Read the model definition and answer for the solid it produces. Units are mm, in the model's axes. Face numbers are marked on the shaded views. A direction names the side the tool comes from. Give positions to 0.01 mm unless a question says otherwise; leave off trailing zeros. Write each loop counter-clockwise with the first axis right and the second up, starting at its lowest first coordinate (ties: lowest second). Pieces come first, ordered by that corner, then holes. Notation, with made-up numbers: M 77.25,8.5 L 119.25,8.5 A13 cw 119.25,27.5 Z; hole C 76,26 d3. An arc over 180 degrees is marked long. Use a Markdown table: item, result. Add a question column.
Item 1: A cutting plane is placed at B-B on x = -7.25. Determine the outline of the cut face in (y, z).
Item 2: Consider probe 1 along Z at (x, y) = (-10.5, 37); probe 2 along X at (y, z) = (36, -1.25); probe 3 along Y at (x, z) = (-5.5, 0.5). Determine where each line is inside the solid, lowest interval first. Write a range as [from, to].
Item 3: A cutting plane is placed at D-D on z = -2.7. Determine the outline of the cut face in (x, y).
Item 4: For the marked faces 1, 2 and 3, determine the directions among +Z, -Z, +X, -X, +Y, -Y from which every point of the face is accessible in a straight line to the end or side of a thin tool.
Item 5: A cutting plane is placed at C-C on y = 35. Determine the outline of the cut face in (x, z).
Item 6: The mould has two halves that part along Y. Classify the marked faces 4, 5, 6 and 7: pulls with the +Y half, pulls with the -Y half, needs draft (parallel to the pull), parting line crosses it, or undercut.
Item 7: A cutting plane is placed at A-A on y = 31.25. Determine the outline of the cut face in (x, z), then the cut area to 3 significant figures.
Item 8: Given P1, Ø1.5, axis at y = 34, z = -1.5, coming from the +X side; P2, Ø1, axis at x = -5.5, z = -2.5, coming from the +Y side; P3, Ø5, axis at x = -7.5, y = 34, coming from the +Z side; P4, Ø2, axis at x = -6.5, z = -1.5, coming from the -Y side, each flat-ended and moving along its own axis, determine where each tip first touches the part or whether it passes through.
from build123d import *

# Parameters (mm, degrees)
SKETCH1_R           = 7
BOSS_EXTRUDE1_DEPTH = 1
SKETCH3_W           = 3
SKETCH3_H           = 10
BOSS_EXTRUDE2_DEPTH = 3
SKETCH5_R           = 2.5
CUT_EXTRUDE1_DEPTH  = 5


with BuildPart() as part:
    # Sketch1 → Boss-Extrude1 (new body)
    with BuildSketch(Plane.XY):
        with Locations((-7.345808821, 32.102080843)):
            Circle(SKETCH1_R)
    extrude(amount=BOSS_EXTRUDE1_DEPTH)

    # Sketch3 → Boss-Extrude2 (add, symmetric)
    with BuildSketch(Plane(origin=(-7.3, 0, 0), x_dir=(0, 0, -1), z_dir=(1, 0, 0))):
        with Locations((1.5, 32.250632967)):
            Rectangle(SKETCH3_W, SKETCH3_H)
    extrude(amount=BOSS_EXTRUDE2_DEPTH, both=True)

    # Sketch5 → Cut-Extrude1 (cut)
    with BuildSketch(Plane.XY.offset(1)):
        with Locations((-7.345808821, 32.102080843)):
            Circle(SKETCH5_R)
    extrude(amount=-CUT_EXTRUDE1_DEPTH, mode=Mode.SUBTRACT)


solid = part.part
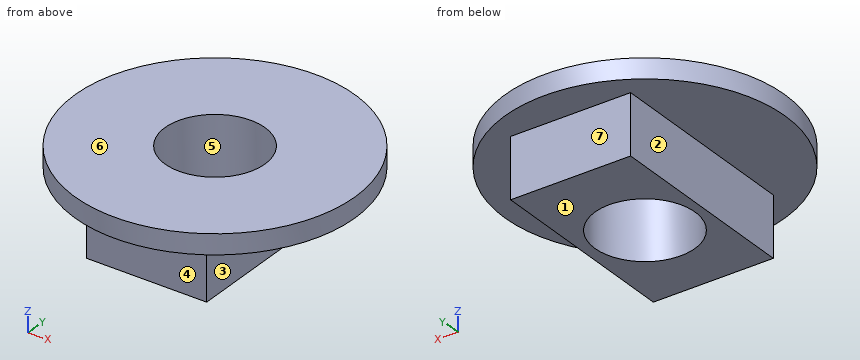
Filled in:
| question | item | result |
|---|---|---|
| 1 | outline | M 25.1,0 L 27.25,0 L 27.25,-3 L 29.6,-3 L 29.6,1 L 25.1,1 Z; M 34.6,-3 L 37.25,-3 L 37.25,0 L 39.1,0 L 39.1,1 L 34.6,1 Z |
| 2 | probe 1 | [0, 1] |
| 2 | probe 2 | [-10.3, -4.3] |
| 2 | probe 3 | [25.35, 30.42], [33.79, 38.85] |
| 3 | outline | M -10.3,27.25 L -4.3,27.25 L -4.3,37.25 L -10.3,37.25 Z; hole C -7.35,32.1 d5 |
| 4 | face 1 | -Z, +X, -X, +Y, -Y |
| 4 | face 2 | -Z, -X, +Y, -Y |
| 4 | face 3 | -Z, +X, +Y, -Y |
| 5 | outline | M -13.72,0 L -10.3,0 L -10.3,-3 L -4.3,-3 L -4.3,0 L -0.97,0 L -0.97,1 L -13.72,1 Z |
| 6 | face 4 | pulls with the -Y half |
| 6 | face 5 | undercut |
| 6 | face 6 | needs draft |
| 6 | face 7 | pulls with the +Y half |
| 7 | outline | M -14.29,0 L -10.3,0 L -10.3,-3 L -9.7,-3 L -9.7,1 L -14.29,1 Z; M -5,-3 L -4.3,-3 L -4.3,0 L -0.4,0 L -0.4,1 L -5,1 Z |
| 7 | area | 13.1 mm² |
| 8 | P1 | x = -4.3 |
| 8 | P2 | y = 37.25 |
| 8 | P3 | z = 1 |
| 8 | P4 | y = 27.25 |
